For this review, take the finished solid that the model builds, in its own axes (mm). Face numbers are marked on the shaded views. A direction names the side the tool comes from. Round coordinates to 2 decimals unless told otherwise and drop trailing zeros. Write each loop counter-clockwise with the first axis right and the second up, starting at its lowest first coordinate (ties: lowest second). Pieces come first, ordered by that corner, then holes. Notation, with made-up numbers: (75, 34.5) - (97, 34.5) arc R36 cw to (97, 72.5) - close; hole circle Ø10 at (-28, 60.5). An arc over 180 degrees is marked (long way). One line per item, written item: value. Start each with the question number.
Q1. Mouldability with a two-part tool opening along Y and no side actions: class the marked faces 3, 4, 5 and 6 as +Y half, -Y half, draft (parallel to the pull), parting line (faces both ways), or undercut.
Q2. Clearance check with flat-ended pins moving along their axes: pin 1 Ø4 at (x, z) = (-27.5, 9) entering from +Y; pin 2 Ø1 at (x, z) = (-14, 8.5) entering from -Y; pin 3 Ø2 at (y, z) = (-25.5, 6.5) entering from -X. State where each tip first meets the part, or that it passes through.
Q3. Tool access review of the marked faces 1 and 2: name each direction out of +Z, -Z, +X, -X, +Y, -Y from which nothing blocks a thin tool from reaching the whole face with its end or side.
Q4. For probe 1 along X at (y, z) = (-7, 4.5); probe 2 along X at (y, z) = (-32, 7); probe 3 along Z at (x, y) = (-62, 9) (3 decimals), list the stretches that pass through material, from the lowest coordinate up.
Q5. Add section C-C on z = 7.5. Write out the cut boundary in (x, y).
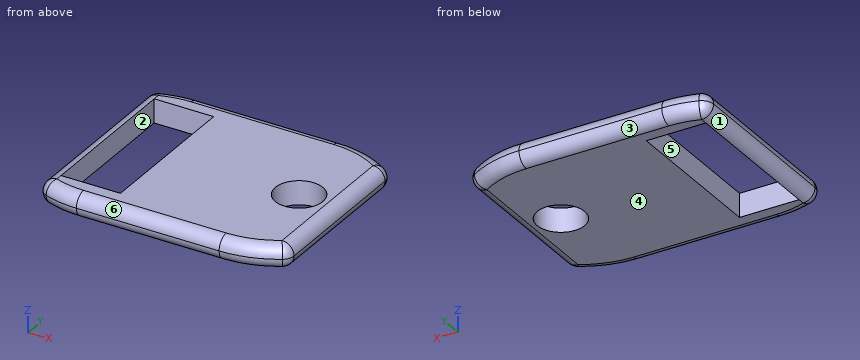
```python
from build123d import *

# Parameters (mm, degrees)
BOSS_EXTRUDE1_DEPTH = 10
SKETCH2_W           = 25
SKETCH2_H           = 65
CUT_EXTRUDE2_DEPTH  = 20
SKETCH3_R           = 10
CUT_EXTRUDE3_DEPTH  = 20
FILLET2_R           = 5


with BuildPart() as part:
    # Sketch1 → Boss-Extrude1 (new body)
    with BuildSketch(Plane.XY):
        with BuildLine():
            Line((-51.324273213, 15.030948404), (8.675726787, 15.030948404))
            ThreePointArc((8.675726787, 15.030948404), (21.820193251, 12.947195155), (33.675726787, 6.900266117))
            Line((33.675726787, 6.900266117), (33.675726787, -61.838369308))
            ThreePointArc((33.675726787, -61.838369308), (21.820193251, -67.885298346), (8.675726787, -69.969051596))
            Line((8.675726787, -69.969051596), (-51.324273213, -69.969051596))
            ThreePointArc((-51.324273213, -69.969051596), (-60.275029546, -69.015819954), (-68.824273213, -66.198885058))
            Line((-68.824273213, -66.198885058), (-68.824273213, 11.260781867))
            ThreePointArc((-68.824273213, 11.260781867), (-60.275029546, 14.077716763), (-51.324273213, 15.030948404))
        make_face()
    extrude(amount=BOSS_EXTRUDE1_DEPTH)

    # Sketch2 → Cut-Extrude2 (cut)
    with BuildSketch(Plane(origin=(0, 0, 0), x_dir=(-1, 0, 0), z_dir=(0, 0, -1))):
        with Locations((51.324273213, -27.469051596)):
            Rectangle(SKETCH2_W, SKETCH2_H)
    extrude(amount=-CUT_EXTRUDE2_DEPTH, mode=Mode.SUBTRACT)

    # Sketch3 → Cut-Extrude3 (cut)
    with BuildSketch(Plane(origin=(0, 0, 0), x_dir=(-1, 0, 0), z_dir=(0, 0, -1))):
        with Locations((-16.675726787, -27.469051596)):
            Circle(SKETCH3_R)
    extrude(amount=-CUT_EXTRUDE3_DEPTH, mode=Mode.SUBTRACT)

    # Fillet2
    fillet2_edges = [part.edges().sort_by_distance(p)[0] for p in [
        (21.820193251, 12.947195155, 10),
        (33.675726787, -27.469051596, 0),
        (21.820193251, -67.885298346, 0),
        (-21.324273213, 15.030948404, 10),
        (8.675726787, -69.969051596, 5),
        (-51.324273213, -69.969051596, 5),
        (-68.824273213, -66.198885058, 5),
        (-68.824273213, 11.260781867, 5),
        (-51.324273213, 15.030948404, 5),
        (8.675726787, 15.030948404, 5),
        (33.675726787, 6.900266117, 5),
        (33.675726787, -61.838369308, 5),
        (-60.275029546, 14.077716763, 10),
        (-68.824273213, -27.469051596, 10),
        (-60.275029546, -69.015819954, 10),
        (-21.324273213, -69.969051596, 10),
        (21.820193251, -67.885298346, 10),
        (33.675726787, -27.469051596, 10),
        (-21.324273213, -69.969051596, 0),
        (-60.275029546, -69.015819954, 0),
        (-68.824273213, -27.469051596, 0),
        (-60.275029546, 14.077716763, 0),
        (-21.324273213, 15.030948404, 0),
        (21.820193251, 12.947195155, 0),
    ]]
    fillet(fillet2_edges, radius=FILLET2_R - 0.0001)  # a hair under: the kernel refuses the full size


solid = part.part
```
Result set:
1. face 3: +Y half
1. face 4: draft
1. face 5: undercut
1. face 6: -Y half
2. pin 1: stops at y = 14.61
2. pin 2: stops at y = -68.97
2. pin 3: stops at x = -68.8
3. face 1: -Z, -X, +Y, -Y
3. face 2: +Z, -Z
4. probe 1: x = -68.8 to -63.82, -38.82 to 33.65
4. probe 2: x = -68.41 to -63.82, -38.82 to 7.76, 25.59 to 33.26
4. probe 3: z = 0.025 to 9.975
5. outline: (-68.15, -62.82) arc R4.33 ccw to (-65.27, -66.91) arc R41.83 ccw to (-51.32, -69.3) - (8.68, -69.3) arc R41.83 ccw to (30.99, -62.85) arc R4.33 ccw to (33.01, -59.19) - (33.01, 4.25) arc R4.33 ccw to (30.99, 7.92) arc R41.83 ccw to (8.68, 14.36) - (-51.32, 14.36) arc R41.83 ccw to (-65.27, 11.97) arc R4.33 ccw to (-68.15, 7.89) - close; hole (-63.82, -59.97) - (-38.82, -59.97) - (-38.82, 5.03) - (-63.82, 5.03) - close; hole circle Ø20 at (16.68, -27.47)
